Source: CAD feature listing. Evaluate the final solid. Frame: model axes, mm. Face numbers are marked on the shaded views. A direction names the side the tool comes from. Give positions to 0.01 mm unless a question says otherwise; leave off trailing zeros. Loops run counter-clockwise (first coordinate to the right, second up) from the corner with the lowest first, then second, coordinate; pieces in that order, holes last. Notation, with made-up numbers: M -22.75,7 L 12.25,7 A22 cw 12.25,15 Z; hole C -20.75,-12.5 d3. An arc over 180 degrees is marked long. Answer in a Markdown table with one row per item.
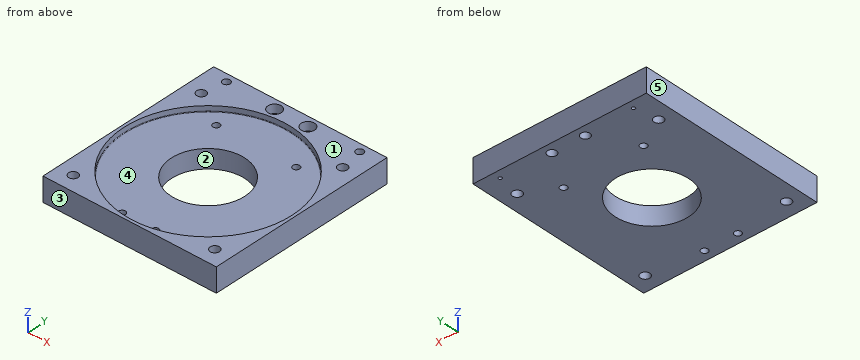
```python
from build123d import *

# Parameters (mm, degrees)
BOSS_EXTRUDE1_DEPTH                                  = 50.8
SKETCH6_W                                            = 7.4
SKETCH6_H                                            = 283
CUT_EXTRUDE3_DEPTH                                   = 306.924238987
SKETCH2_R                                            = 126
CUT_EXTRUDE1_DEPTH                                   = 8
M16_TAPPED_HOLE1_D                                   = 14
SKETCH5_R                                            = 55
CUT_EXTRUDE2_DEPTH                                   = 203.714084365
FILLET1_R                                            = 0.79375
CBORE_FOR_M12_HEX_SOCKET_HEAD_CAP_SCREW1_D           = 13.5
CBORE_FOR_M12_HEX_SOCKET_HEAD_CAP_SCREW1_CBORE_D     = 20
CBORE_FOR_M12_HEX_SOCKET_HEAD_CAP_SCREW1_CBORE_DEPTH = 13
M12_TAPPED_HOLE1_D                                   = 10.2
M6_TAPPED_HOLE1_D                                    = 5
M6_TAPPED_HOLE1_DEPTH                                = 27.99
M6_TAPPED_HOLE1_TIP                                  = 1.502151548
F_11_2_11_2_DIAMETER_HOLE1_D                         = 11.2
F_11_2_11_2_DIAMETER_HOLE1_DEPTH                     = 20
F_11_2_11_2_DIAMETER_HOLE1_TIP                       = 3.364819467


with BuildPart() as part:
    # Sketch1 → Boss-Extrude1 (new body)
    with BuildSketch(Plane.XY):
        Polygon((-130, 130), (-130, -130), (130, -130), (130, 130), (130, 153), (-130, 153), align=None)
    extrude(amount=BOSS_EXTRUDE1_DEPTH)

    # Sketch6 → Cut-Extrude3 (cut, through all)
    with BuildSketch(Plane(origin=(130, 0, 0), x_dir=(0, 0, -1), z_dir=(1, 0, 0))):
        with Locations((-3.7, 11.5)):
            Rectangle(SKETCH6_W, SKETCH6_H)
        with Locations((-47.1, 11.5)):
            Rectangle(SKETCH6_W, SKETCH6_H)
    extrude(amount=-CUT_EXTRUDE3_DEPTH, mode=Mode.SUBTRACT)

    # Sketch2 → Cut-Extrude1 (cut)
    with BuildSketch(Plane.XY.offset(43.4)):
        Circle(SKETCH2_R)
    extrude(amount=-CUT_EXTRUDE1_DEPTH, mode=Mode.SUBTRACT)

    # M16 Tapped Hole1 (through all)
    with Locations(Plane(origin=(116.1053078, 120.483553204, 43.4), x_dir=(1, 0, 0), z_dir=(0, 0, 1))):
        with Locations((-222.171324978, -14.417536026), (-10.039290622, -14.417536026), (-10.039290622, -226.549570382), (-222.171324978, -226.549570382)):
            Hole(M16_TAPPED_HOLE1_D / 2)

    # Sketch5 → Cut-Extrude2 (cut, through all)
    with BuildSketch(Plane.XY.offset(35.4)):
        Circle(SKETCH5_R)
    extrude(amount=-CUT_EXTRUDE2_DEPTH, mode=Mode.SUBTRACT)

    # Fillet1
    fillet1_edges = [part.edges().sort_by_distance(p)[0] for p in [
        (-126, 0, 35.4),
    ]]
    fillet(fillet1_edges, radius=FILLET1_R)

    # CBORE for M12 Hex Socket Head Cap Screw1 (through all)
    with Locations(Plane.XY.offset(43.4)):
        with Locations((-25, 138), (25, 138)):
            CounterBoreHole(CBORE_FOR_M12_HEX_SOCKET_HEAD_CAP_SCREW1_D / 2, CBORE_FOR_M12_HEX_SOCKET_HEAD_CAP_SCREW1_CBORE_D / 2, CBORE_FOR_M12_HEX_SOCKET_HEAD_CAP_SCREW1_CBORE_DEPTH)

    # M12 Tapped Hole1 (through all)
    with Locations(Plane(origin=(0, 0, 7.4), x_dir=(-1, 0, 0), z_dir=(0, 0, -1))):
        with Locations((-60, 80), (60, 80), (25, -115), (-25, -115)):
            Hole(M12_TAPPED_HOLE1_D / 2)

    # M6 Tapped Hole1
    with Locations(Plane(origin=(0, 0, 7.4), x_dir=(-1, 0, 0), z_dir=(0, 0, -1))):
        with Locations((100, 141), (-100, 141)):
            Hole(M6_TAPPED_HOLE1_D / 2, depth=M6_TAPPED_HOLE1_DEPTH)
            with Locations((0, 0, -(M6_TAPPED_HOLE1_DEPTH + M6_TAPPED_HOLE1_TIP / 2))):  # 118° drill point
                Cone(0, M6_TAPPED_HOLE1_D / 2, M6_TAPPED_HOLE1_TIP, mode=Mode.SUBTRACT)

    # Ø11.2 (11.2) Diameter Hole1
    with Locations(Plane.XY.offset(43.4)):
        with Locations((100, 141), (-100, 141)):
            Hole(F_11_2_11_2_DIAMETER_HOLE1_D / 2, depth=F_11_2_11_2_DIAMETER_HOLE1_DEPTH)
            with Locations((0, 0, -(F_11_2_11_2_DIAMETER_HOLE1_DEPTH + F_11_2_11_2_DIAMETER_HOLE1_TIP / 2))):  # 118° drill point
                Cone(0, F_11_2_11_2_DIAMETER_HOLE1_D / 2, F_11_2_11_2_DIAMETER_HOLE1_TIP, mode=Mode.SUBTRACT)


solid = part.part
```
1) Pull-direction query (Y, two-part tool) for the marked faces 1, 2 and 3; classes: released by +Y, released by -Y, zero draft, split by the parting line, or undercut.
Reply:
| item | result |
|---|---|
| face 1 | zero draft |
| face 2 | undercut |
| face 3 | released by -Y |
2) Section A-A, the plane x = 0. Return loops of the section in (y, z), then the cut area to 3 significant figures.
Reply:
| item | result |
|---|---|
| outline | M -130,7.4 L -55,7.4 L -55,35.4 L -125.21,35.4 A0.79 cw -126,36.19 L -126,43.4 L -130,43.4 Z; M 55,7.4 L 153,7.4 L 153,43.4 L 126,43.4 L 126,36.19 A0.79 cw 125.21,35.4 L 55,35.4 Z |
| area | 5,090 mm² |
3) Material intervals for L1, parallel to X at y = -1, z = 33; L2, parallel to X at y = 141, z = 36.5; L3, parallel to X at y = 76.5, z = 29, sorted ascending.
Reply:
| item | result |
|---|---|
| L1 | x = -130 to -54.99, 54.99 to 130 |
| L2 | x = -130 to -105.6, -94.4 to -34.54, -15.46 to 15.46, 34.54 to 94.4, 105.6 to 130 |
| L3 | x = -130 to -63.71, -56.29 to 56.29, 63.71 to 130 |
4) Section B-B, the plane z = 13. Count the separate pieces of the cut face and the enclosed holes in it, then the cut area to 3 significant figures.
Reply:
| item | result |
|---|---|
| separate pieces | 1 |
| enclosed holes | 13 |
| area | 62,800 mm² |
5) Set-up query: the marked faces 4 and 5. Return all of +Z, -Z, +X, -X, +Y, -Y with unobstructed straight access to the full face (end or side cutting, diameter ignored); none if empty.
Reply:
| item | result |
|---|---|
| face 4 | +Z |
| face 5 | +Z, -Z, -X, +Y, -Y |
6) Pin query (flat end, axial travel): pin 1 Ø10 at (x, y) = (-74.5, 49) entering from +Z; pin 2 Ø16 at (x, y) = (-25, 138) entering from +Z; pin 3 Ø8 at (x, y) = (100, 141) entering from +Z. Return the tip coordinate at first contact, or that it passes through.
Reply:
| item | result |
|---|---|
| pin 1 | stops at z = 35.4 |
| pin 2 | stops at z = 30.4 |
| pin 3 | stops at z = 22.44 |
